Read the model definition and answer for the solid it produces. Units are mm, in the model's axes. Coordinates: 2 decimals unless noted, no trailing zeros. Loops run counter-clockwise (first coordinate to the right, second up) from the corner with the lowest first, then second, coordinate; pieces in that order, holes last. Notation, with made-up numbers: (67.25, 48) - (101.25, 48) arc R13 cw to (101.25, 58) - close; hole circle Ø11 at (68.25, 20). An arc over 180 degrees is marked (long way). Use CSV: the item, a comma, the result in double quotes.
Autodesk Inventor part; units mm, degrees
ref_plane "РабПлоскость2" through (-8.3726, 0, 0) normal (1, 0, 0) x (0, 0, -1)
ref_plane "YZ Plane" through (0, 0, 0) normal (1, 0, 0) x (0, 1, 0)
ref_plane "XZ Plane" through (0, 0, 0) normal (0, 1, 0) x (-1, 0, 0)
sketch "Эскиз1" plane through (0, 0, 0) normal (0, 0, 1) x (1, 0, 0)
  line L0 (0, 0) -> (-8.3726, 0)
  arc A0 (-6, 1.9227) -> (-8, 2.2534) centre (-7.0273, 1.9227) ccw
  line L1 (-6, 1.9227) -> (-6, 1.45)
  line L2 (-6, 1.45) -> (0, 1.45)
  line L3 (0, 1.45) -> (0, 0)
  line L4 (-8.6724, 2.95) -> (-6.1128, 2.95)
  arc A1 (-8, 2.2534) -> (-8.3726, 0) centre (-1.3726, 0) ccw
  dimension "d0" = 2.9
  dimension "d1" = 5.9
  dimension "d2" = 2
  dimension "d3" = 6
  dimension "d4" = 7
revolve "Вращение1" add sketch "Эскиз1" angle 360 about axis through (0, 0, 0) along (-1, 0, 0)
chamfer "Фаска1" distance 0.3 angle 45 1 edges at (0, -1.45, 0)
ref_plane "РабПлоскость2" through (-8.3726, 0, 0) normal (1, 0, 0) x (0, 0, -1)
sketch "Эскиз2" plane through (-8.3726, 0, 0) normal (1, 0, 0) x (0, 0, -1)
  line L0 (-0.4, 1.5) -> (0.4, 1.5)
  line L1 (0.4, 1.5) -> (0.4, -1.5)
  line L2 (0.4, -1.5) -> (-0.4, -1.5)
  line L3 (-0.4, -1.5) -> (-0.4, 1.5)
  line L4 (-1.5, 0.4) -> (1.5, 0.4)
  line L5 (1.5, 0.4) -> (1.5, -0.4)
  line L6 (1.5, -0.4) -> (-1.5, -0.4)
  line L7 (-1.5, -0.4) -> (-1.5, 0.4)
  point P0 (0, 0)
  point P1 (0, 1.5)
  point P2 (0, 0.4)
  point P3 (-1.5, 0)
  point P4 (-0.4, 0)
  point P5 (0.4, 0.4)
  point P6 (-0.4, 0.4)
  point P7 (-0.4, -0.4)
  point P8 (0.4, -0.4)
  dimension "d10" = 0.8
  dimension "d11" = 3
extrude "Выдавливание1" cut sketch "Эскиз2" along normal blind 1.2
properties part number "Винт М3х19"
Q1. The part is cut by section A-A on x = -3.5. Determine the outline of the cut face in (y, z).
Reported:
outline,"circle Ø2.9 at (0, 0)"
Q2. For a pull along Z with two mould halves and no side action, classify faces 1 (the face through (-3.11, -1.45, 0.06)), 2 (the face through (-8, 1, -0.4)), 3 (the face through (0, 0, 0)) as +Z half, -Z half, draft (parallel to the pull), parting line (faces both ways), or undercut.
Reported:
face 1,"parting line"
face 2,"undercut"
face 3,"draft"
Q3. Find the intervals of material crossed by probe 1 along X at (y, z) = (1.1, 0.1); probe 2 along Y at (x, z) = (-2.75, 0.05); probe 3 along X at (y, z) = (0.95, -1.45), in increasing order. Write a range as [from, to].
Reported:
probe 1,"x = [-7.17, 0]"
probe 2,"y = [-1.45, 1.45]"
probe 3,"x = [-8.15, -6]"
Q4. Given P1, Ø0.6, axis at x = -7.5, z = 0, coming from the +Y side; P2, Ø1.2, axis at x = -8, y = -1, coming from the -Z side; P3, Ø1.2, axis at x = -8, z = 1, coming from the -Y side, each flat-ended and moving along its own axis, determine where each tip first touches the part or whether it passes through.
Reported:
P1,"stops at y = 2.94"
P2,"stops at z = -2.76"
P3,"stops at y = -2.76"
Q5. The part is cut by section B-B on x = -6.25. Determine the outline of the cut face in (y, z), and give its area (3 significant figures).
Reported:
outline,"circle Ø5.19 at (0, 0)"
area,"21.1 mm²"
